Source: CAD feature listing. Evaluate the final solid. Frame: model axes, mm. Round coordinates to 2 decimals unless told otherwise and drop trailing zeros. Loops run counter-clockwise (first coordinate to the right, second up) from the corner with the lowest first, then second, coordinate; pieces in that order, holes last. Notation, with made-up numbers: M 35,51.25 L 56,51.25 A24 cw 56,71.25 Z; hole C -12.5,28.25 d5. An arc over 180 degrees is marked long. Answer as a JSON object with one key per item and string values.
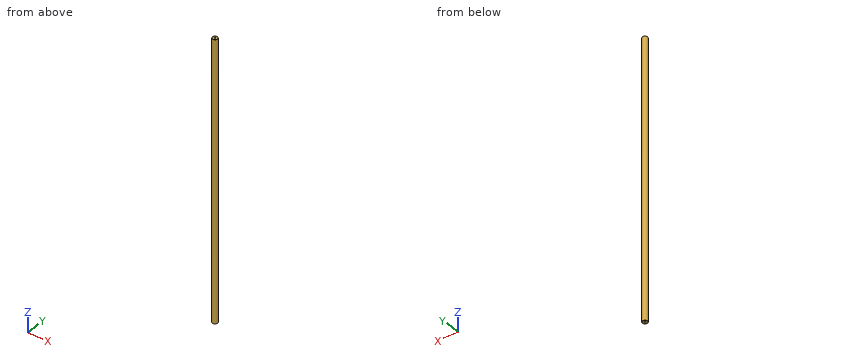
Autodesk Inventor part; units mm, degrees
ref_plane "YZ Plane" through (0, 0, 0) normal (1, 0, 0) x (0, 1, 0)
ref_plane "XZ Plane" through (0, 0, 0) normal (0, 1, 0) x (-1, 0, 0)
ref_plane "XY Plane" through (0, 0, 0) normal (0, 0, 1) x (1, 0, 0)
sketch "Sketch1" plane through (0, 0, 0) normal (0, 0, 1) x (1, 0, 0)
  circle A0 centre (-28, -169.4449) radius 2
  circle A1 centre (-28, -169.4449) radius 5
  point P0 (0, 0)
  dimension "d0" = 10
extrude "Extrusion1" add sketch "Sketch1" along normal blind 533 contours A0 | A1
sketch "Sketch2" plane through (-28, -169.4449, 533) normal (0, 0, 1) x (1, 0, 0)
  circle A0 centre (0, 0) radius 5
  point P0 (28, 169.4449)
hole "Hole1" at (-28, -169.4449, 533) direction (0, 0, -1) diameter 3.242 depth 17 tip angle 118
sketch "Sketch3" plane through (-28, -169.4449, 0) normal (0, 0, -1) x (-1, 0, 0)
  circle A0 centre (0, 0) radius 5
  point P0 (-28, 169.4449)
hole "Hole2" at (-28, -169.4449, 0) direction (0, 0, 1) diameter 3.242 depth 17 tip angle 118
chamfer "Chamfer1" distance 0.2 angle 45 2 edges at (-33, -169.4449, 0) (-33, -169.4449, 533)
properties material "Stainless Steel"
Item 1: Line query: probe 1 along Y at (x, z) = (-28, 524.5); probe 2 along X at (y, z) = (-170.25, 477); probe 3 along X at (y, z) = (-168, 449.5). Output: solid intervals per line, ascending. Write a range as from..to.
Answer sheet:
{"probe 1": "y = -174.44..-171.07, -167.82..-164.44", "probe 2": "x = -32.93..-23.07", "probe 3": "x = -32.79..-23.21"}
Item 2: Contact query for flat-ended pins moving along their axis: pin 1 Ø1.5 at (y, z) = (-171.5, 269) entering from +X; pin 2 Ø3 at (x, y) = (-28, -169.44) entering from +Z; pin 3 Ø5 at (x, z) = (-31.5, 470) entering from +Y. Output: stop coordinate, or through.
Answer sheet:
{"pin 1": "stops at x = -23.17", "pin 2": "stops at z = 515.93", "pin 3": "stops at y = -164.55"}
Item 3: Section A-A on z = 54. Return the cut outline in (x, y).
Answer sheet:
{"outline": "C -28,-169.44 d10"}
